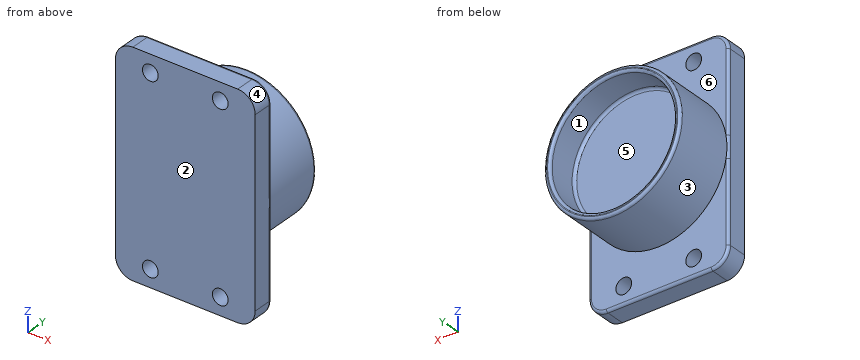
from build123d import *

# Parameters (mm, degrees)
SZKIC1_W                    = 80
SZKIC1_H                    = 125
DODANIE_WYCI_GNI_CIE1_DEPTH = 12
SZKIC2_R                    = 39
SZKIC2_R_2                  = 35.5
DODANIE_WYCI_GNI_CIE2_DEPTH = 35
SZKIC4_R                    = 35.5
DODANIE_WYCI_GNI_CIE3_DEPTH = 17
ZAOKR_GLENIE1_R             = 10
ZAOKR_GLENIE2_R             = 1.5


with BuildPart() as part:
    # Szkic1 → Dodanie-wyciągnięcie1 (new body)
    with BuildSketch(Plane(origin=(0, 0, 0), x_dir=(1, 0, 0), z_dir=(0, 1, 0))):
        Rectangle(SZKIC1_W, SZKIC1_H)
    extrude(amount=DODANIE_WYCI_GNI_CIE1_DEPTH)

    # Szkic2 → Dodanie-wyciągnięcie2 (add)
    with BuildSketch(Plane(origin=(0, 12, 0), x_dir=(1, 0, 0), z_dir=(0, 1, 0))):
        with Locations(Location((0, 0, 0), (0, 0, 270))):
            Circle(SZKIC2_R)
        with Locations(Location((0, 0, 0), (0, 0, 270))):
            Circle(SZKIC2_R_2, mode=Mode.SUBTRACT)
    extrude(amount=DODANIE_WYCI_GNI_CIE2_DEPTH)

    # Szkic4 → Dodanie-wyciągnięcie3 (add)
    with BuildSketch(Plane(origin=(0, 12, 0), x_dir=(1, 0, 0), z_dir=(0, 1, 0))):
        with Locations(Location((0, 0, 0), (0, 0, 270))):
            Circle(SZKIC4_R)
    extrude(amount=DODANIE_WYCI_GNI_CIE3_DEPTH)

    # Zaokrąglenie1
    zaokr_glenie1_edges = [part.edges().sort_by_distance(p)[0] for p in [
        (-40, 6, -62.5),
        (40, 6, -62.5),
        (40, 6, 62.5),
        (-40, 6, 62.5),
    ]]
    fillet(zaokr_glenie1_edges, radius=ZAOKR_GLENIE1_R)

    # Zaokrąglenie2
    zaokr_glenie2_edges = [part.edges().sort_by_distance(p)[0] for p in [
        (0, 47, -39),
        (0, 47, -35.5),
        (0, 29, -35.5),
        (0, 12, -62.5),
        (40, 12, 0),
        (-40, 12, 0),
        (0, 12, 62.5),
        (37.071067812, 12, 59.571067812),
        (-37.071067812, 12, 59.571067812),
        (-37.071067812, 12, -59.571067812),
        (37.071067812, 12, -59.571067812),
    ]]
    fillet(zaokr_glenie2_edges, radius=ZAOKR_GLENIE2_R)

    # Szkic9 → Otwór pod śrubę M82 (revolve, cut)
    with BuildSketch(Plane(origin=(-20, 12, 52.5), x_dir=(0, 0, 1), z_dir=(1, 0, 0))):
        Polygon((0, 0), (0, 18.703872786), (4.5, 16), (4.5, 0), align=None)
    otw_r_pod_rub_m82 = revolve(axis=Axis((-20, 18.35, 52.5), (0, -1, 0)), mode=Mode.SUBTRACT)

    # Lustro3: Otwór pod śrubę M82 across plane
    add(otw_r_pod_rub_m82.mirror(Plane(origin=(0, 0, 0), x_dir=(0, 0, 1), z_dir=(1, 0, 0))), mode=Mode.SUBTRACT)

    # Lustro4: Otwór pod śrubę M82 across plane
    add(otw_r_pod_rub_m82.mirror(Plane.XY), mode=Mode.SUBTRACT)

    # Lustro4 copy 1 sketch → Lustro4 copy 1 (revolve, cut)
    with BuildSketch(Plane(origin=(20, 12, -52.5), x_dir=(0, 0, -1), z_dir=(-1, 0, 0))):
        Polygon((0, 0), (0, 18.703872786), (4.5, 16), (4.5, 0), align=None)
    revolve(axis=Axis((20, 18.35, -52.5), (0, -1, 0)), mode=Mode.SUBTRACT)


solid = part.part
Verification items for the finished model (mm, model axes). Face numbers are marked on the shaded views. A direction names the side the tool comes from. Coordinates: 2 decimals unless noted, no trailing zeros. Order: outer loops, then holes, each group sorted by start corner. A loop starts at its lowest first (then second) coordinate and runs counter-clockwise, first axis right, second up. Notation, with made-up numbers: (-35, 87.5) -> (-22, 87.5) arc R12 ccw to (-22, 109.5) -> close; hole circle Ø5 at (88.25, -17). An arc over 180 degrees is marked (long way). Use CSV: the item, a comma, the result in double quotes. Start each with the question number.
Q1. Draft check along Z on the marked faces 3, 4, 5 and 6. Enter one of: +Z half, -Z half, draft (parallel to the pull), parting line (faces both ways), or undercut.
Q2. Section check C-C, the plane y = 43. Record the cut outline in (x, z), and give its area (3 significant figures).
Q3. Thickness scan on line 1 along Z through (x, y) = (-20, 7.5); line 2 along X through (y, z) = (4, -52); line 3 along X through (y, z) = (38.25, 0). Record the ranges inside material, lowest first.
Q4. Section check B-B, the plane x = 0. Record the cut outline in (y, z).
Q5. Section check A-A, the plane z = -45. Record the cut outline in (x, y).
Q6. Depth check by flat-ended pin: P1, Ø6, axis at y = 14, z = 5.5, coming from the +X side; P2, Ø14.5, axis at x = -20, z = -52.5, coming from the +Y side; P3, Ø5, axis at x = -0.5, z = -14, coming from the +Y side. Enter the tip coordinate at first touch or a pass-through.
Q7. Tool access check on the marked faces 1 and 2. Record the directions out of +Z, -Z, +X, -X, +Y, -Y that give a thin tool (end or side, any length) a straight path to the whole face; none if there is none.
Q8. Section check D-D, the plane x = 20. Give the number of separate pieces and of enclosed holes in the cut face, and give its area (3 significant figures).
Returned:
1,face 3,"parting line"
1,face 4,"+Z half"
1,face 5,"undercut"
1,face 6,"draft"
2,outline,"circle Ø78 at (0, 0); hole circle Ø71 at (0, 0)"
2,area,"819 mm^2"
3,line 1,"z = -62.5 to -57, -48 to 48, 57 to 62.5"
3,line 2,"x = -40 to -24.47, -15.53 to 15.53, 24.47 to 40"
3,line 3,"x = -39 to -35.5, 35.5 to 39"
4,outline,"(0, -62.5) -> (10.5, -62.5) arc R1.5 ccw to (12, -61) -> (12, -39) -> (45.5, -39) arc R1.5 ccw to (47, -37.5) -> (47, -37) arc R1.5 ccw to (45.5, -35.5) -> (30.5, -35.5) arc R1.5 cw to (29, -34) -> (29, 34) arc R1.5 cw to (30.5, 35.5) -> (45.5, 35.5) arc R1.5 ccw to (47, 37) -> (47, 37.5) arc R1.5 ccw to (45.5, 39) -> (12, 39) -> (12, 61) arc R1.5 ccw to (10.5, 62.5) -> (0, 62.5) -> close"
5,outline,"(-40, 0) -> (40, 0) -> (40, 10.5) arc R1.5 ccw to (38.5, 12) -> (-38.5, 12) arc R1.5 ccw to (-40, 10.5) -> close"
6,P1,"stops at x = 39.92"
6,P2,"stops at y = 12"
6,P3,"stops at y = 29"
7,face 1,"+Y"
7,face 2,"+Z, -Z, +X, -X, -Y"
8,separate pieces,"3"
8,enclosed holes,"0"
8,area,"2,570 mm^2"
